Here's the drawing with two shaded views (mm, measured from the low corner). I have some questions. A direction names the side the tool comes from. Round coordinates to 2 decimals unless told otherwise and drop trailing zeros. Order: outer loops, then holes, each group sorted by start corner. A loop starts at its lowest first (then second) coordinate and runs counter-clockwise, first axis right, second up. Notation, with made-up numbers: (-31, 1.5) -> (-2, 1.5) arc R21 ccw to (-2, 5.5) -> close; hole circle Ø9 at (41.5, -4). An arc over 180 degrees is marked (long way). Use a Markdown table: item, result. Add a question column.
Q1. I'm going to push flat-ended pins straight in: pin 1 Ø1.8 at (x, z) = (9, 3.5) entering from +Y; pin 2 Ø2 at (x, z) = (3, 6) entering from +Y; pin 3 Ø2.5 at (x, z) = (19, 5.5) entering from -Y; pin 4 Ø8 at (x, y) = (8, 15) entering from -Z. Where does each tip first touch, or does it pass through?
Q2. We'd pull the mould along X, two halves only. Please class the marked faces 5, 6, 7 and 8: +X half, -X half, draft (parallel to the pull), parting line (faces both ways), or undercut.
Q3. If we section it at D-D on x = 4: List the corners of the cut face in (y, z) for me.
Q4. I need wall thicknesses on line 1 along Y through (x, z) = (20.2, 5); line 2 along Y through (x, z) = (2.5, 0.5); line 3 along X through (y, z) = (42.5, 7). Which ranges of each line are inside material? Lowest first, please. Write a range as [from, to].
Q5. If we section it at C-C on y = 63.5: List the corners of the cut face in (x, z) for me (1 decimal).
Q6. For the marked faces 1, 2, 3 and 4, which set-ups out of +Z, -Z, +X, -X, +Y, -Y let a thin tool reach every point of the face, with its end or its side?
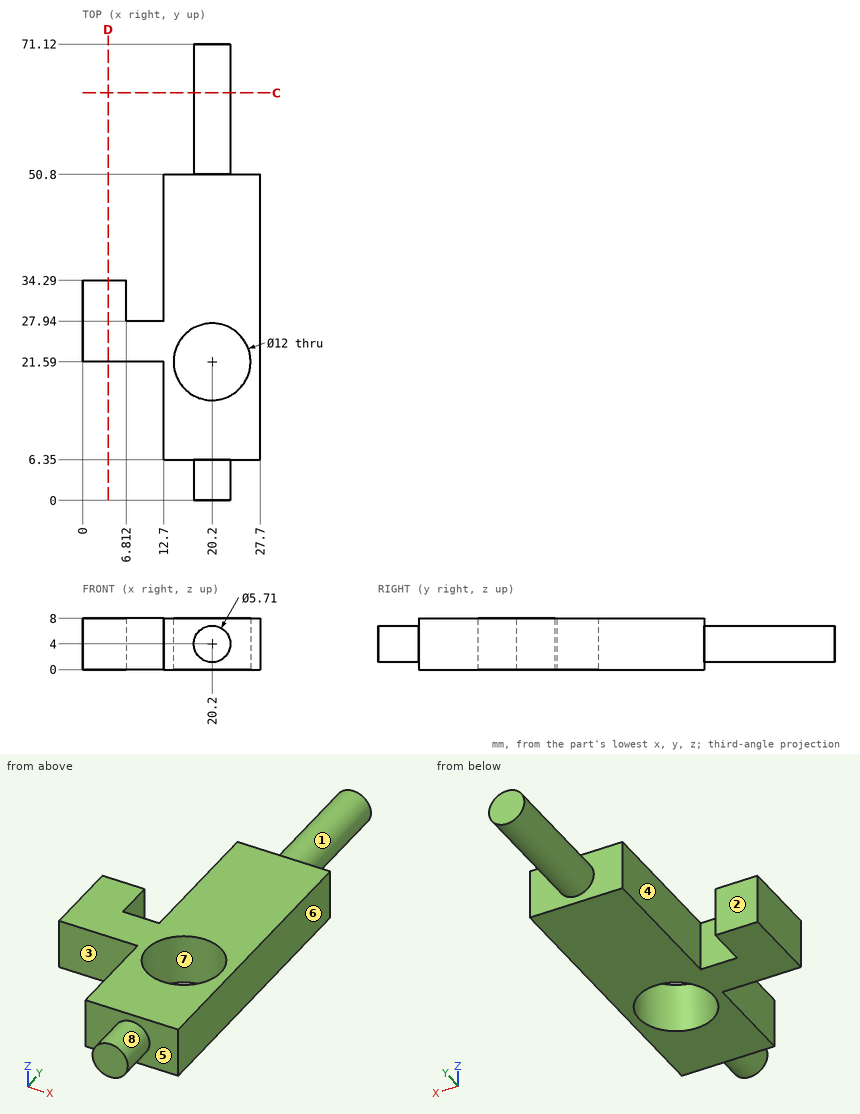
Answer below:
| question | item | result |
|---|---|---|
| 1 | pin 1 | y = 27.94 |
| 1 | pin 2 | y = 34.29 |
| 1 | pin 3 | y = 0 |
| 1 | pin 4 | through |
| 2 | face 5 | draft |
| 2 | face 6 | +X half |
| 2 | face 7 | undercut |
| 2 | face 8 | parting line |
| 3 | outline | (21.59, 0) -> (34.29, 0) -> (34.29, 8) -> (21.59, 8) -> close |
| 4 | line 1 | [0, 15.59], [27.59, 71.12] |
| 4 | line 2 | [21.59, 34.29] |
| 4 | line 3 | [12.7, 27.7] |
| 5 | outline | circle Ø5.7 at (20.2, 4) |
| 6 | face 1 | +Y |
| 6 | face 2 | +Z, -Z, -X, +Y |
| 6 | face 3 | +Z, -Z, -X, -Y |
| 6 | face 4 | +Z, -Z, +Y |
